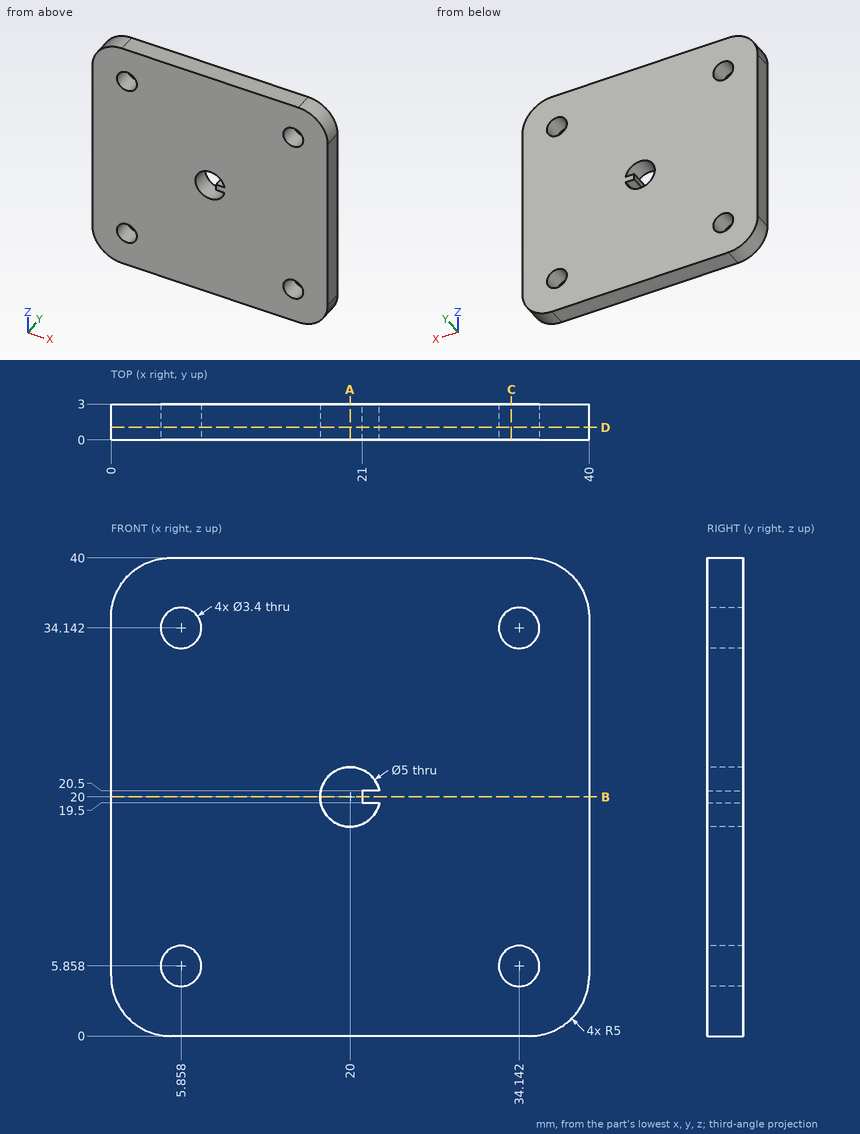
For this review, use the dimensioned drawing (mm, ordinates from the lowest corner) and the shaded views. Give positions to 0.01 mm unless a question says otherwise; leave off trailing zeros. Order: outer loops, then holes, each group sorted by start corner. A loop starts at its lowest first (then second) coordinate and runs counter-clockwise, first axis right, second up. Notation, with made-up numbers: (27.25, 32.5) - (36.25, 32.5) arc R20 ccw to (36.25, 55.5) - close; hole circle Ø5 at (-35, 25). An arc over 180 degrees is marked (long way). Use a Markdown table: item, result. Add a question column.
(1) Wall thickness on probe 1 along X at (y, z) = (2.35, 20); probe 2 along Z at (x, y) = (33, 1.75); probe 3 along X at (y, z) = (2.05, 35): over which ranges is each line inside the solid? List them lowest first. Write a range as [from, to].
(2) Add section A-A on x = 20. Give the boundary of the cut face in (y, z), then the cut area to 3 significant figures.
(3) Add section C-C on x = 33.5. Give the boundary of the cut face in (y, z), then the cut area to 3 significant figures.
(4) Add section D-D on y = 1.05. Give the boundary of the cut face in (x, z).
(5) Add section B-B on z = 20. Give the boundary of the cut face in (x, y), then the cut area to 4 significant figures.
Report:
| question | item | result |
|---|---|---|
| 1 | probe 1 | x = [0, 17.5], [21, 40] |
| 1 | probe 2 | z = [0, 4.6], [7.12, 32.88], [35.4, 40] |
| 1 | probe 3 | x = [0, 4.39], [7.33, 32.67], [35.61, 40] |
| 2 | outline | (0, 0) - (3, 0) - (3, 17.5) - (0, 17.5) - close; (0, 22.5) - (3, 22.5) - (3, 40) - (0, 40) - close |
| 2 | area | 105 mm² |
| 3 | outline | (0, 0) - (3, 0) - (3, 4.28) - (0, 4.28) - close; (0, 7.43) - (3, 7.43) - (3, 32.57) - (0, 32.57) - close; (0, 35.72) - (3, 35.72) - (3, 40) - (0, 40) - close |
| 3 | area | 101 mm² |
| 4 | outline | (0, 5) arc R5 ccw to (5, 0) - (35, 0) arc R5 ccw to (40, 5) - (40, 35) arc R5 ccw to (35, 40) - (5, 40) arc R5 ccw to (0, 35) - close; hole circle Ø3.4 at (5.86, 5.86); hole circle Ø3.4 at (5.86, 34.14); hole (21, 19.5) - (21, 20.5) - (22.45, 20.5) arc R2.5 ccw (long way) to (22.45, 19.5) - close; hole circle Ø3.4 at (34.14, 5.86); hole circle Ø3.4 at (34.14, 34.14) |
| 5 | outline | (0, 0) - (17.5, 0) - (17.5, 3) - (0, 3) - close; (21, 0) - (40, 0) - (40, 3) - (21, 3) - close |
| 5 | area | 109.5 mm² |
